Check sheet for the modelled part. Datum: model origin and axes. Units: mm. A direction names the side the tool comes from. Round coordinates to 2 decimals unless told otherwise and drop trailing zeros. Write each loop counter-clockwise with the first axis right and the second up, starting at its lowest first coordinate (ties: lowest second). Pieces come first, ordered by that corner, then holes. Notation, with made-up numbers: (29.25, 42) - (67.25, 42) arc R30 cw to (67.25, 75) - close; hole circle Ø2 at (84.5, 38). An arc over 180 degrees is marked (long way). Answer as a JSON object with one key per item and string values. Group by question number.
Item 1: Sectioned sample at B-B on z = -18. Record the boundary of the cut face in (x, y) (3 decimals).
Item 2: Thickness scan on line 1 (Y direction, x = -12.75, z = -27); line 2 (Y direction, x = -16.25, z = -21); line 3 (Z direction, x = -6, y = -0.5). Record the ranges inside material, lowest first.
Item 3: Sectioned sample at D-D on y = 94. Record the boundary of the cut face in (x, z) (3 decimals).
Item 4: Set-up check for faces 1 (the cylindrical face through (-8.8, 117.1, -23.9)), 2 (the flat face through (-3.175, 59, -24)), 3 (the flat face through (-7, 45, -6.35)): record each of +Z, -Z, +X, -X, +Y, -Y from which the full face is reachable in a straight line by a thin tool's end or side.
Item 5: Sectioned sample at A-A on y = 114. Record the boundary of the cut face in (x, z) (3 decimals).
Item 6: Gauge pin test, flat ends, axial feed: P1, Ø1.5, axis at x = -6, y = 73, coming from the +Z side; P2, Ø15.5, axis at y = 108.99, z = -20.57, coming from the +X side; P3, Ø3, axis at y = 39.5, z = -3, coming from the +X side. Record the tip position at first contact, or that the pin passes through.
Item 7: Release check for a two-part mould opening along Y. For faces 4 (the flat face through (-11, -29.12, -19)), 5 (the flat face through (-13, 61, 6.35)), 6 (the cylindrical face through (-7.765, 78.648, 0.089)) record: pulls with the +Y half, pulls with the -Y half, needs draft (parallel to the pull), parting line crosses it, or undercut.
```python
from build123d import *

# Parameters (mm, degrees)
BOSS_EXTRUDE1_DEPTH = 6.35
FILLET1_R           = 3.175
SKETCH3_W           = 16.2814
SKETCH3_H           = 177.8
BOSS_EXTRUDE2_DEPTH = 38.1
SKETCH4_R           = 6.7437
CUT_EXTRUDE1_DEPTH  = 157.034307273
SKETCH5_R           = 8.7641176
CUT_EXTRUDE2_DEPTH  = 11.3284


with BuildPart() as part:
    # Sketch1 → Boss-Extrude1 (new, symmetric)
    with BuildSketch(Plane.XY):
        with BuildLine():
            Line((-3.175, 148.680256121), (-19.4564, 148.680256121))
            Line((-19.4564, 148.680256121), (-19.4564, -29.119743879))
            Line((-19.4564, -29.119743879), (-3.175, -29.119743879))
            Line((-3.175, -29.119743879), (-3.175, -13.930255965))
            ThreePointArc((-3.175, -13.930255965), (-11.533104962, -8.433276125), (-14.237180291, 1.198062439))
            Line((-14.237180291, 1.198062439), (-7.84751395, 77.129690658))
            ThreePointArc((-7.84751395, 77.129690658), (-7.764904905, 78.669797764), (-7.775922348, 80.212079439))
            Line((-7.775922348, 80.212079439), (-9.518300378, 126.6428125))
            ThreePointArc((-9.518300378, 126.6428125), (-7.878891544, 132.352447387), (-3.175, 135.980256121))
            Line((-3.175, 135.980256121), (-3.175, 148.680256121))
        make_face()
    extrude(amount=BOSS_EXTRUDE1_DEPTH, both=True)

    # Fillet1
    fillet1_edges = [part.edges().sort_by_distance(p)[0] for p in [
        (-3.175, 135.980256121, 0),
        (-3.175, -13.930255965, 0),
    ]]
    fillet(fillet1_edges, radius=FILLET1_R)

    # Sketch3 → Boss-Extrude2 (add)
    with BuildSketch(Plane(origin=(0, 0, -6.35), x_dir=(-1, 0, 0), z_dir=(0, 0, -1))):
        with Locations((11.3157, 59.780256121)):
            Rectangle(SKETCH3_W, SKETCH3_H)
    extrude(amount=BOSS_EXTRUDE2_DEPTH)

    # Sketch4 → Cut-Extrude1 (cut, through all)
    with BuildSketch(Plane(origin=(-3.175, 0, 0), x_dir=(0, 0, -1), z_dir=(1, 0, 0))):
        with Locations(Location((20.574, 108.991994121, 0), (0, 0, 90))):
            Circle(SKETCH4_R)
        with Locations(Location((20.574, 10.568518121, 0), (0, 0, 90))):
            Circle(SKETCH4_R)
    extrude(amount=-CUT_EXTRUDE1_DEPTH, mode=Mode.SUBTRACT)

    # Sketch5 → Cut-Extrude2 (cut)
    with BuildSketch(Plane(origin=(-3.175, 0, 0), x_dir=(0, 0, -1), z_dir=(1, 0, 0))):
        with Locations(Location((20.574, 108.991994121, 0), (0, 0, 90))):
            Circle(SKETCH5_R)
        with Locations(Location((20.574, 10.568518121, 0), (0, 0, 90))):
            Circle(SKETCH5_R)
    extrude(amount=-CUT_EXTRUDE2_DEPTH, mode=Mode.SUBTRACT)


solid = part.part
```
Completed:
{
 "1": {"outline": "(-19.456, -29.12) - (-3.175, -29.12) - (-3.175, 2.191) - (-14.503, 2.191) - (-14.503, 4.335) - (-19.456, 4.335) - close; (-19.456, 16.802) - (-14.503, 16.802) - (-14.503, 18.946) - (-3.175, 18.946) - (-3.175, 100.614) - (-14.503, 100.614) - (-14.503, 102.759) - (-19.456, 102.759) - close; (-19.456, 115.225) - (-14.503, 115.225) - (-14.503, 117.37) - (-3.175, 117.37) - (-3.175, 148.68) - (-19.456, 148.68) - close"},
 "2": {"line 1": "-29.12 to 4.61, 16.53 to 103.03, 114.95 to 148.68", "line 2": "-29.12 to 3.84, 17.3 to 102.26, 115.72 to 148.68", "line 3": "-44.45 to -6.35"},
 "3": {"outline": "(-19.456, -44.45) - (-3.175, -44.45) - (-3.175, -6.35) - (-8.293, -6.35) - (-8.293, 6.35) - (-19.456, 6.35) - close"},
 "4": {"face 1": "+X", "face 2": "+Z, -Z, +X, +Y, -Y", "face 3": "+Z, +X"},
 "5": {"outline": "(-19.456, -44.45) - (-3.175, -44.45) - (-3.175, -27.766) - (-14.503, -27.766) - (-14.503, -25.09) - (-19.456, -25.09) - close; (-19.456, -16.058) - (-14.503, -16.058) - (-14.503, -13.382) - (-3.175, -13.382) - (-3.175, -6.35) - (-9.044, -6.35) - (-9.044, 6.35) - (-19.456, 6.35) - close"},
 "6": {"P1": "z = -6.35", "P2": "x = -14.5", "P3": "x = -10.89"},
 "7": {"face 4": "pulls with the -Y half", "face 5": "needs draft", "face 6": "undercut"}
}
